CAD build for the part. Positions are in the model's coordinates, mm. Face numbers are marked on the shaded views. A direction names the side the tool comes from. Give positions to 0.01 mm unless a question says otherwise; leave off trailing zeros. Loops run counter-clockwise (first coordinate to the right, second up) from the corner with the lowest first, then second, coordinate; pieces in that order, holes last. Notation, with made-up numbers: (78.5, 41) - (120.5, 41) arc R25 cw to (120.5, 79) - close; hole circle Ø3 at (78, 69.5). An arc over 180 degrees is marked (long way). Return JSON: item names as keys, results as strings.
from build123d import *

# Parameters (mm, degrees)
SKETCH1_W           = 120
SKETCH1_H           = 75
SKETCH1_R           = 3
BOSS_EXTRUDE1_DEPTH = 10
SKETCH2_R           = 2.5
CUT_EXTRUDE1_DEPTH  = 7
SKETCH3_R           = 1.5
CUT_EXTRUDE2_DEPTH  = 10
LPATTERN1_COUNT     = 2
LPATTERN1_PITCH     = 110
SKETCH4_W           = 120
SKETCH4_H           = 130
BOSS_EXTRUDE2_DEPTH = 10
SKETCH5_R           = 1.5
CUT_EXTRUDE3_DEPTH  = 10
LPATTERN2_COUNT     = 2
LPATTERN2_PITCH     = 110


with BuildPart() as part:
    # Sketch1 → Boss-Extrude1 (new body)
    with BuildSketch(Plane.XY):
        Rectangle(SKETCH1_W, SKETCH1_H)
        with Locations((-44, 31.5)):
            Circle(SKETCH1_R, mode=Mode.SUBTRACT)
        with Locations((44, 31.5)):
            Circle(SKETCH1_R, mode=Mode.SUBTRACT)
        with Locations((-44, -31.5)):
            Circle(SKETCH1_R, mode=Mode.SUBTRACT)
        with Locations((44, -31.5)):
            Circle(SKETCH1_R, mode=Mode.SUBTRACT)
    extrude(amount=BOSS_EXTRUDE1_DEPTH)

    # Sketch2 → Cut-Extrude1 (cut)
    with BuildSketch(Plane.XY.offset(10)):
        with Locations((0, 10)):
            Circle(SKETCH2_R)
        with Locations((0, -10)):
            Circle(SKETCH2_R)
    extrude(amount=-CUT_EXTRUDE1_DEPTH, mode=Mode.SUBTRACT)

    # Sketch3 → Cut-Extrude2 (cut)
    with BuildSketch(Plane(origin=(60, 0, 0), x_dir=(0, 0, -1), z_dir=(1, 0, 0))):
        with Locations(Location((-5, 17.5, 0), (0, 0, 90))):
            Circle(SKETCH3_R)
        with Locations(Location((-5, -17.5, 0), (0, 0, 90))):
            Circle(SKETCH3_R)
    cut_extrude2 = extrude(amount=-CUT_EXTRUDE2_DEPTH, mode=Mode.SUBTRACT)

    # LPattern1: Cut-Extrude2 ×2
    with Locations(*[(-i * LPATTERN1_PITCH, 0, 0) for i in range(1, LPATTERN1_COUNT)]):
        add(cut_extrude2, mode=Mode.SUBTRACT)

    # Sketch4 → Boss-Extrude2 (add)
    with BuildSketch(Plane(origin=(0, 37.5, 0), x_dir=(1, 0, 0), z_dir=(0, 1, 0))):
        with Locations((0, -50)):
            Rectangle(SKETCH4_W, SKETCH4_H)
    extrude(amount=BOSS_EXTRUDE2_DEPTH)

    # Sketch5 → Cut-Extrude3 (cut)
    with BuildSketch(Plane(origin=(60, 0, 0), x_dir=(0, 0, -1), z_dir=(1, 0, 0))):
        with Locations(Location((-105, 42.5, 0), (0, 0, 90))):
            Circle(SKETCH5_R)
        with Locations(Location((-25, 42.5, 0), (0, 0, 90))):
            Circle(SKETCH5_R)
    cut_extrude3 = extrude(amount=-CUT_EXTRUDE3_DEPTH, mode=Mode.SUBTRACT)

    # LPattern2: Cut-Extrude3 ×2
    with Locations(*[(-i * LPATTERN2_PITCH, 0, 0) for i in range(1, LPATTERN2_COUNT)]):
        add(cut_extrude3, mode=Mode.SUBTRACT)


solid = part.part
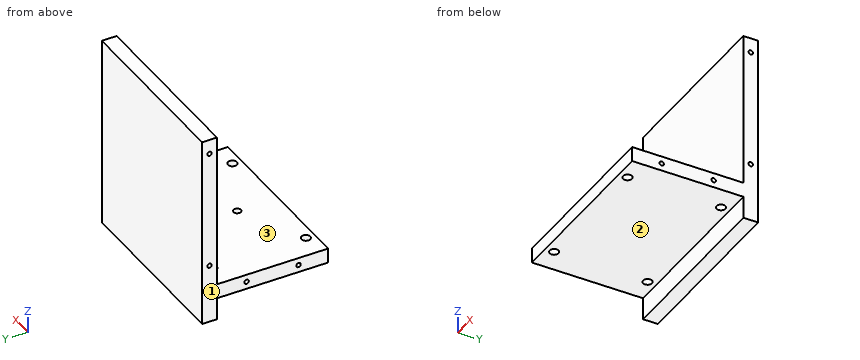
1. Drop flat-ended pins along their axis: P1, Ø4, axis at y = 42.5, z = 105, coming from the +X side; P2, Ø5, axis at x = 44, y = 31.5, coming from the -Z side; P3, Ø1.5, axis at y = 43, z = 105, coming from the -X side; P4, Ø1.5, axis at x = 12.5, y = -21, coming from the -Z side. Give the stop position or say it passes through.
Values follow:
{"P1": "stops at x = 60", "P2": "passes through", "P3": "stops at x = -50", "P4": "stops at z = 0"}
2. Which spindle directions (+Z, -Z, +X, -X, +Y, -Y) get a long thin tool onto all of the face, cutting with end or side? Do the marked faces 1, 2 and 3. Say none if no direction does.
Values follow:
{"face 1": "+Z, -Z, -X, +Y, -Y", "face 2": "-Z, +X, -X, -Y", "face 3": "+Z, +X, -X, -Y"}
3. Drill centre lines: probe 1 along Z at (x, y) = (-56, 42.5); probe 2 along Y at (x, z) = (26.5, 57.5); probe 3 along Z at (x, y) = (14, -17.5). Where is each one in solid material? Low to high.
Values follow:
{"probe 1": "z = -15 to 23.5, 26.5 to 103.5, 106.5 to 115", "probe 2": "y = 37.5 to 47.5", "probe 3": "z = 0 to 10"}
4. Cut at D-D, the plane z = 29.5. Write the cut outline in (x, y), plus the area to 3 significant figures.
Values follow:
{"outline": "(-60, 37.5) - (60, 37.5) - (60, 47.5) - (-60, 47.5) - close", "area": "1,200 mm²"}
5. Cut at C-C, the plane x = 0. Write the cut outline in (y, z).
Values follow:
{"outline": "(-37.5, 0) - (37.5, 0) - (37.5, -15) - (47.5, -15) - (47.5, 115) - (37.5, 115) - (37.5, 10) - (12.5, 10) - (12.5, 3) - (7.5, 3) - (7.5, 10) - (-7.5, 10) - (-7.5, 3) - (-12.5, 3) - (-12.5, 10) - (-37.5, 10) - close"}
6. Cut at B-B, the plane x = -44. Write the cut outline in (y, z), plus the area to 3 significant figures.
Values follow:
{"outline": "(-37.5, 0) - (-34.5, 0) - (-34.5, 10) - (-37.5, 10) - close; (-28.5, 0) - (28.5, 0) - (28.5, 10) - (-28.5, 10) - close; (34.5, 0) - (37.5, 0) - (37.5, -15) - (47.5, -15) - (47.5, 115) - (37.5, 115) - (37.5, 10) - (34.5, 10) - close", "area": "1,930 mm²"}
7. Cut at A-A, the plane y = 31.5. Write the cut outline in (x, z), plus the area to 3 significant figures.
Values follow:
{"outline": "(-60, 0) - (-47, 0) - (-47, 10) - (-60, 10) - close; (-41, 0) - (41, 0) - (41, 10) - (-41, 10) - close; (47, 0) - (60, 0) - (60, 10) - (47, 10) - close", "area": "1,080 mm²"}
